Answer from the drawing. Dimensions are ordinates in mm from the lowest x, y and z of the part. A direction names the side the tool comes from. Round coordinates to 2 decimals unless told otherwise and drop trailing zeros. Write each loop counter-clockwise with the first axis right and the second up, starting at its lowest first coordinate (ties: lowest second). Pieces come first, ordered by that corner, then holes. Notation, with made-up numbers: (59, -6.5) - (72, -6.5) arc R9 cw to (72, -0.5) - close; hole circle Ø8 at (29, 43.5). An arc over 180 degrees is marked (long way). Use a Markdown table: item, result. Add a question column.
1) A tool of negligible diameter and unlimited length cuts with its end or side. For the marked faces 1 and 2, from which of +Z, -Z, +X, -X, +Y, -Y can it reach the whole face along a straight path? Write none if from no direction.
2) A cutting plane is placed at B-B (z = 15). Give the vertices of the cut face in (x, y).
3) A cutting plane is placed at C-C (y = 10.5). Give the vertices of the cut face in (x, z), then the cut area to 3 significant figures.
4) This flat-tipped pin is pushed along its axis until it touches: P1, Ø3, axis at x = 12, y = 1.5, coming from the -Z side. Where does it stop, or does it pass through?
5) A cutting plane is placed at A-A (z = 30.5). Give the vertices of the cut face in (x, y).
6) Find the intervals of material crossed by probe 1 along X at (y, z) = (4, 10.5) (1 decimal); probe 2 along Z at (x, y) = (11.5, 6.5); probe 3 along X at (y, z) = (4.25, 25.5) (1 decimal), in increasing order. Write a range as from..to.
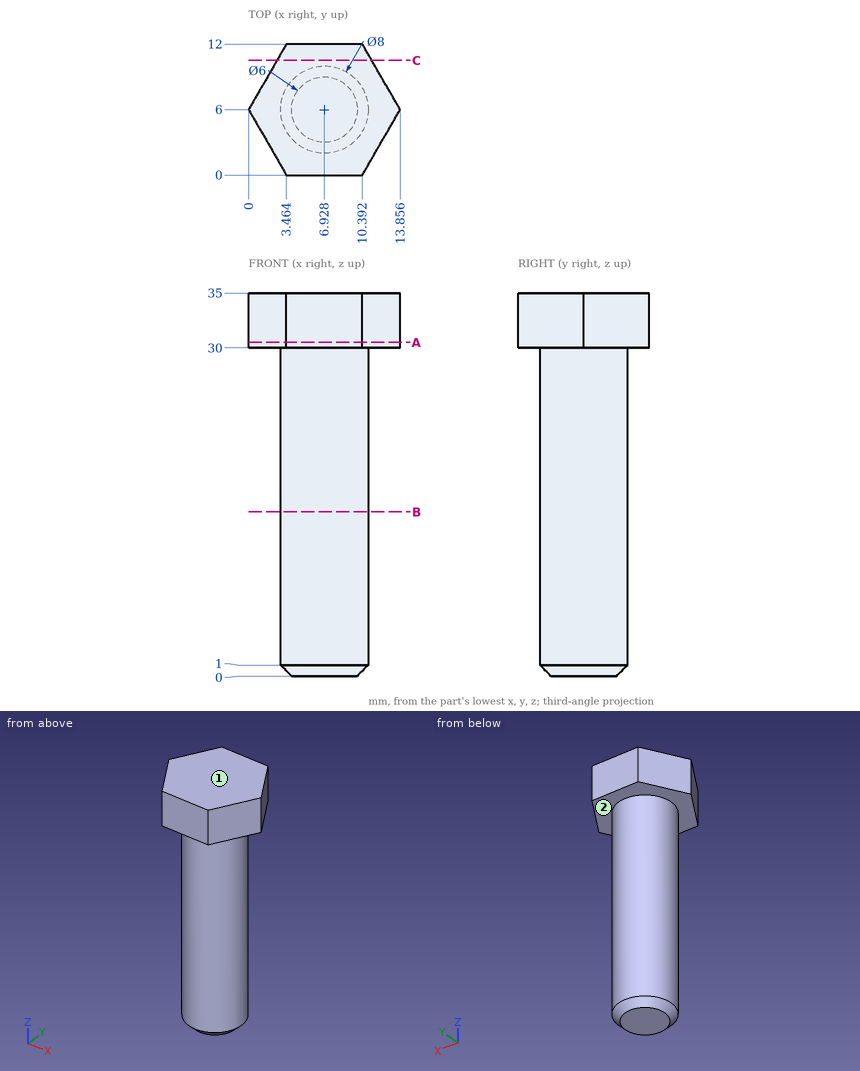
Entries:
| question | item | result |
|---|---|---|
| 1 | face 1 | +Z, +X, -X, +Y, -Y |
| 1 | face 2 | -Z |
| 2 | outline | circle Ø8 at (6.93, 6) |
| 3 | outline | (2.6, 30) - (11.26, 30) - (11.26, 35) - (2.6, 35) - close |
| 3 | area | 43.3 mm² |
| 4 | P1 | stops at z = 30 |
| 5 | outline | (0, 6) - (3.46, 0) - (10.39, 0) - (13.86, 6) - (10.39, 12) - (3.46, 12) - close |
| 6 | probe 1 | x = 3.5..10.4 |
| 6 | probe 2 | z = 30..35 |
| 6 | probe 3 | x = 3.3..10.5 |
